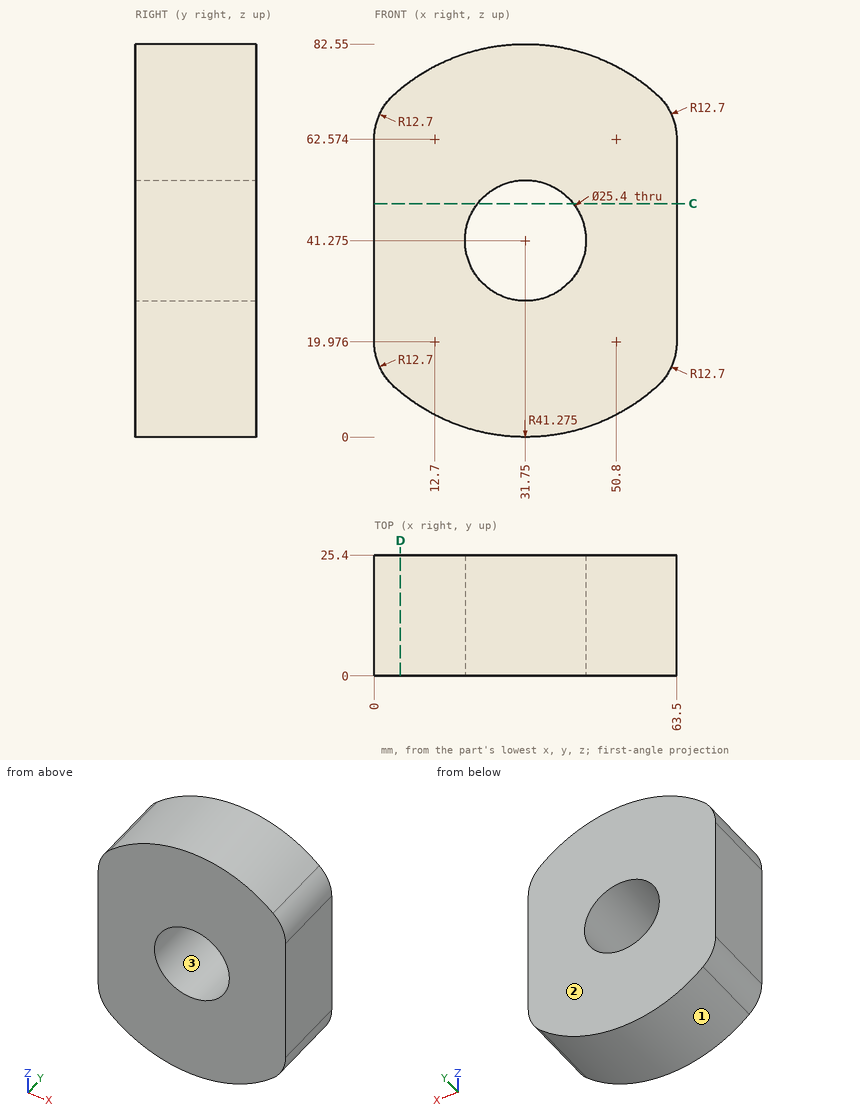
Could you check a few things on this drawing? It's one solid part, dimensions in mm from its lowest x, y, z. Coordinates: 2 decimals unless noted, no trailing zeros. Write each loop counter-clockwise with the first axis right and the second up, starting at its lowest first coordinate (ties: lowest second). Pieces come first, ordered by that corner, then holes.
Q1. Imagine slicing it at D-D, the plane x = 5.5. List the corners of the cut face in (y, z) for me, plus the area to 3 significant figures.
Results found:
outline: (0, 9.42) - (25.4, 9.42) - (25.4, 73.13) - (0, 73.13) - close
area: 1,620 mm2
Q2. Imagine slicing it at C-C, the plane z = 49. List the corners of the cut face in (x, y) for me, plus the area to 3 significant figures.
Results found:
outline: (0, 0) - (21.67, 0) - (21.67, 25.4) - (0, 25.4) - close; (41.83, 0) - (63.5, 0) - (63.5, 25.4) - (41.83, 25.4) - close
area: 1,100 mm2
Q3. Please list where these lines run through material, in increasing order: L1, parallel to Z at x = 37.5, y = 13.25; L2, parallel to Z at x = 43.5, y = 15 (1 decimal); L3, parallel to X at y = 5, z = 40.5.
Results found:
L1: z = 0.4 to 29.95, 52.6 to 82.15
L2: z = 1.7 to 36.5, 46.1 to 80.8
L3: x = 0 to 19.07, 44.43 to 63.5
Q4. For P1, Ø2, axis at x = 51.5, y = 19.5, coming from the -Z side (1 decimal), with a flat end and sliding along its axis, tell me the tip position at first contact or that it passes through.
Results found:
P1: stops at z = 4.5
Q5. If we mould it in two halves opening along Z, with no side actions, what happens to the marked faces 1, 2 and 3? For each: +Z half, -Z half, draft (parallel to the pull), parting line (faces both ways), or undercut.
Results found:
face 1: -Z half
face 2: draft
face 3: undercut
